```python
from build123d import *

# Parameters (mm, degrees)
SKETCH_1_W          = 10
SKETCH_1_H          = 9.6
SKETCH_1_R          = 2
SKETCH_1_W_2        = 9.6
SKETCH_1_H_2        = 10
SKETCH_1_R_2        = 4
EXTRUDE_2_DEPTH     = 3
SKETCH_2_R          = 3.95
EXTRUDE_3_DEPTH     = 120
CUT_EXTRUDE_START   = -60
SKETCH_3_R          = 3.95
CUT_EXTRUDE_1_DEPTH = 60
SKETCH_4_R          = 4.95
EXTRUDE_4_DEPTH     = 60


with BuildPart() as part:
    # 草图1 → 凸台-拉伸2 (new body)
    # profile 1 of 6: a face of its own
    with BuildSketch(Plane(origin=(0, 0, 0), x_dir=(1, 0, 0), z_dir=(0, 1, 0))):
        with Locations((-9.8, 0)):
            Rectangle(SKETCH_1_W, SKETCH_1_H)
        with Locations(Location((-9.946440474, 0.053559526, 0), (0, 0, 270))):
            Circle(SKETCH_1_R, mode=Mode.SUBTRACT)
    # profile 2 of 6: a face of its own
    with BuildSketch(Plane(origin=(0, 0, 0), x_dir=(1, 0, 0), z_dir=(0, 1, 0))):
        with Locations((0, -9.8)):
            Rectangle(SKETCH_1_W_2, SKETCH_1_H_2)
        with Locations(Location((-0.053559526, -9.946440474, 0), (0, 0, 270))):
            Circle(SKETCH_1_R, mode=Mode.SUBTRACT)
    # profile 3 of 6: a face of its own
    with BuildSketch(Plane(origin=(0, 0, 0), x_dir=(1, 0, 0), z_dir=(0, 1, 0))):
        Rectangle(SKETCH_1_W_2, SKETCH_1_H)
        Circle(SKETCH_1_R_2, mode=Mode.SUBTRACT)
    # profile 4 of 6: a face of its own
    with BuildSketch(Plane(origin=(0, 0, 0), x_dir=(1, 0, 0), z_dir=(0, 1, 0))):
        with Locations((9.8, 0)):
            Rectangle(SKETCH_1_W, SKETCH_1_H)
        with Locations(Location((9.946440474, -0.053559526, 0), (0, 0, 270))):
            Circle(SKETCH_1_R, mode=Mode.SUBTRACT)
    # profile 5 of 6: a face of its own
    with BuildSketch(Plane(origin=(0, 0, 0), x_dir=(1, 0, 0), z_dir=(0, 1, 0))):
        with Locations((0, 9.8)):
            Rectangle(SKETCH_1_W_2, SKETCH_1_H_2)
        with Locations(Location((0.053559526, 9.946440474, 0), (0, 0, 270))):
            Circle(SKETCH_1_R, mode=Mode.SUBTRACT)
    # profile 6 of 6: a face of its own
    with BuildSketch(Plane(origin=(0, 0, 0), x_dir=(1, 0, 0), z_dir=(0, 1, 0))):
        Circle(SKETCH_1_R_2)
    extrude(amount=EXTRUDE_2_DEPTH)

    # 草图2 → 凸台-拉伸3 (add)
    with BuildSketch(Plane(origin=(0, 3, 0), x_dir=(1, 0, 0), z_dir=(0, 1, 0))):
        with Locations(Location((0, 0, 0), (0, 0, 270))):
            Circle(SKETCH_2_R)
    extrude(amount=EXTRUDE_3_DEPTH)

    # 草图3 → 切除-拉伸1 (cut)
    with BuildSketch(Plane(origin=(0, 123, 0), x_dir=(1, 0, 0), z_dir=(0, 1, 0)).offset(CUT_EXTRUDE_START)):
        with Locations(Location((0, 0, 0), (0, 0, 270))):
            Circle(SKETCH_3_R)
    extrude(amount=CUT_EXTRUDE_1_DEPTH, mode=Mode.SUBTRACT)

    # 草图4 → 凸台-拉伸4 (add)
    with BuildSketch(Plane(origin=(0, 63, 0), x_dir=(1, 0, 0), z_dir=(0, 1, 0))):
        with Locations(Location((0, 0, 0), (0, 0, 270))):
            Circle(SKETCH_4_R)
    extrude(amount=-EXTRUDE_4_DEPTH)


solid = part.part
```
Here's how the part is built. I have some questions about the finished solid (model axes, mm). A direction names the side the tool comes from. Coordinates: 2 decimals unless noted, no trailing zeros. Order: outer loops, then holes, each group sorted by start corner. A loop starts at its lowest first (then second) coordinate and runs counter-clockwise, first axis right, second up.
1) Imagine slicing it at D-D on y = 13. List the corners of the cut face in (x, z) for me.
2) We'd pull the mould along Z, two halves only. Please class faces 4 (the face through (4.8, 1, 10)), 5 (the face through (0, 1, -14.8)), 6 (the face through (1.49, 33.42, 4.72)), 7 (the face through (-1.27, 1.48, 8.36)): +Z half, -Z half, draft (parallel to the pull), parting line (faces both ways), or undercut.
3) I need wall thicknesses on line 1 (Y direction, x = -8.5, z = -4.5); line 2 (Z direction, x = -1.25, y = 42.5); line 3 (X direction, y = 10, z = -0.25). Which ranges of each line are inside material? Lowest first, please.
4) Which directions (+Z, -Z, +X, -X, +Y, -Y) give clear straight access to the entire face, cutting with the end or side of a thin tool? Please do faces 1 (the face through (-4.8, 1, 10)), 2 (the face through (10, 1, -4.8)), 3 (the face through (-10, 1, -4.8)).
5) Imagine slicing it at A-A on z = 0. List the corners of the cut face in (x, y) for me.
6) Imagine slicing it at B-B on z = -10.25. List the corners of the cut face in (x, y) for me.
7) Imagine slicing it at C-C on z = -3.5. List the corners of the cut face in (x, y) for me, and give its area (3 significant figures).
8) Will these pins go through, and if not, where does the flat tip stop? pin 1 (3.5 mm diameter, centred on y = 2, z = -11.5, fed in from +X); pin 2 (1.5 mm diameter, centred on x = -7.5, y = 1.5, fed in from +Z); pin 3 (3.5 mm diameter, centred on y = 1.5, z = -11, fed in from -X).
Response values:
1. outline: circle Ø9.9 at (0, 0)
2. face 4: draft
2. face 5: -Z half
2. face 6: parting line
2. face 7: undercut
3. line 1: y = 0 to 3
3. line 2: z = -4.79 to 4.79
3. line 3: x = -4.94 to 4.94
4. face 1: +Z, -X, +Y, -Y
4. face 2: -Z, +X, +Y, -Y
4. face 3: -Z, -X, +Y, -Y
5. outline: (-14.8, 0) - (-11.95, 0) - (-11.95, 3) - (-14.8, 3) - close; (-7.95, 0) - (7.95, 0) - (7.95, 3) - (4.95, 3) - (4.95, 63) - (-4.95, 63) - (-4.95, 3) - (-7.95, 3) - close; (11.95, 0) - (14.8, 0) - (14.8, 3) - (11.95, 3) - close
6. outline: (-4.8, 0) - (-1.92, 0) - (-1.92, 3) - (-4.8, 3) - close; (2.03, 0) - (4.8, 0) - (4.8, 3) - (2.03, 3) - close
7. outline: (-14.8, 0) - (14.8, 0) - (14.8, 3) - (3.5, 3) - (3.5, 63) - (-3.5, 63) - (-3.5, 3) - (-14.8, 3) - close
7. area: 509 mm2
8. pin 1: stops at x = 4.8
8. pin 2: stops at z = 4.8
8. pin 3: stops at x = -4.8
